Geometry check sheet. Reference: the model listing, model coordinates, mm. Face numbers are marked on the shaded views. A direction names the side the tool comes from. Give positions to 0.01 mm unless a question says otherwise; leave off trailing zeros. Write each loop counter-clockwise with the first axis right and the second up, starting at its lowest first coordinate (ties: lowest second). Pieces come first, ordered by that corner, then holes. Notation, with made-up numbers: (47, 81.25) - (90, 81.25) arc R7 ccw to (90, 86.25) - close; hole circle Ø2 at (36.5, 24.25). An arc over 180 degrees is marked (long way). Write item = value, one per line. Start each with the question number.
(1) Section check B-B, the plane y = -12. Enter the section's corners in (x, z), plus the area to 3 significant figures.
(2) Section check C-C, the plane z = 3. Enter the section's corners in (x, y).
(3) Section check A-A, the plane z = -10. Enter the section's corners in (x, y), plus the area to 3 significant figures.
(4) Access from +Z, -Z, +X, -X, +Y, -Y to the whole of each face (thin tool, end or side, straight path). Record for the marked faces 5 and 6.
(5) Draft check along X on the marked faces 1, 2, 3 and 4. Enter one of: pulls with the +X half, pulls with the -X half, needs draft (parallel to the pull), parting line crosses it, or undercut.
(6) Depth check by flat-ended pin: pin 1 Ø1.5 at (x, z) = (-1.5, -11) entering from +Y; pin 2 Ø8 at (x, y) = (8, 2) entering from -Z; pin 3 Ø4 at (x, z) = (10, -10) entering from +Y. Enter the tip coordinate at first touch or a pass-through.
(7) Thickness scan on L1, parallel to Z at x = -10, y = -12; L2, parallel to Z at x = 6.5, y = 2.25; L3, parallel to Y at x = -9, z = -14. Record the ranges inside material, lowest first.
(8) Section check D-D, the plane y = 0.75. Enter the section's corners in (x, z).
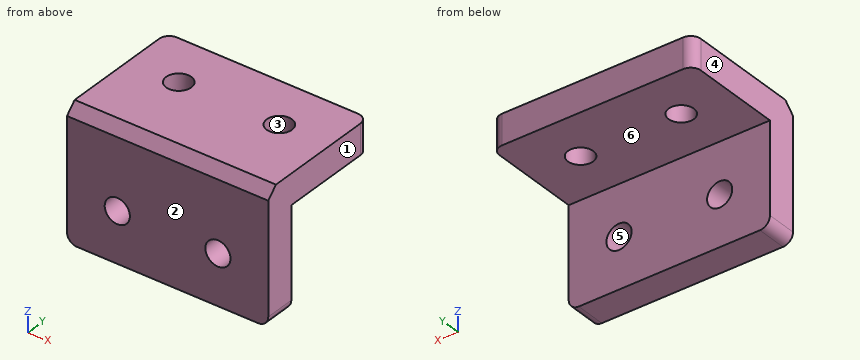
```python
from build123d import *

# Parameters (mm, degrees)
SKETCH1_R           = 2.5
BOSS_EXTRUDE2_DEPTH = 6
SKETCH3_W           = 40
SKETCH3_H           = 6
BOSS_EXTRUDE3_DEPTH = 26
SKETCH4_R           = 2.5
CUT_EXTRUDE2_DEPTH  = 26
CHAMFER1_SIZE       = 2


with BuildPart() as part:
    # Sketch1 → Boss-Extrude2 (new body)
    with BuildSketch(Plane.XY):
        with BuildLine():
            Line((-20, -9.25), (20, -9.25))
            Line((20, -9.25), (20, 8.75))
            ThreePointArc((20, 8.75), (19.414213562, 10.164213562), (18, 10.75))
            Line((18, 10.75), (-18, 10.75))
            ThreePointArc((-18, 10.75), (-19.414213562, 10.164213562), (-20, 8.75))
            Line((-20, 8.75), (-20, -9.25))
        make_face()
        with Locations((-10, 0.75)):
            Circle(SKETCH1_R, mode=Mode.SUBTRACT)
        with Locations((10, 0.75)):
            Circle(SKETCH1_R, mode=Mode.SUBTRACT)
    extrude(amount=BOSS_EXTRUDE2_DEPTH)

    # Sketch3 → Boss-Extrude3 (add)
    with BuildSketch(Plane.XY.offset(6)):
        with Locations((0, -12.25)):
            Rectangle(SKETCH3_W, SKETCH3_H)
    extrude(amount=-BOSS_EXTRUDE3_DEPTH)

    # Sketch4 → Cut-Extrude2 (cut)
    with BuildSketch(Plane.XZ.offset(15.25)):
        with Locations((-10, -10)):
            Circle(SKETCH4_R)
        with Locations((10, -10)):
            Circle(SKETCH4_R)
        with BuildLine():
            Line((-20, -20), (-18, -20))
            ThreePointArc((-18, -20), (-19.414213562, -19.414213562), (-20, -18))
            Line((-20, -18), (-20, -20))
        make_face()
        with BuildLine():
            ThreePointArc((20, -18), (19.414213562, -19.414213562), (18, -20))
            Line((18, -20), (20, -20))
            Line((20, -20), (20, -18))
        make_face()
    extrude(amount=-CUT_EXTRUDE2_DEPTH, mode=Mode.SUBTRACT)

    # Chamfer1
    chamfer1_edges = [part.edges().sort_by_distance(p)[0] for p in [
        (0, -15.25, 6),
    ]]
    chamfer(chamfer1_edges, length=CHAMFER1_SIZE)


solid = part.part
```
Model answer:
q1.outline = (-20, -18) arc R2 ccw to (-18, -20) - (18, -20) arc R2 ccw to (20, -18) - (20, 6) - (-20, 6) - close; hole circle Ø5 at (-10, -10); hole circle Ø5 at (10, -10)
q1.area = 999 mm²
q2.outline = (-20, -15.25) - (20, -15.25) - (20, 8.75) arc R2 ccw to (18, 10.75) - (-18, 10.75) arc R2 ccw to (-20, 8.75) - close; hole circle Ø5 at (-10, 0.75); hole circle Ø5 at (10, 0.75)
q3.outline = (-20, -15.25) - (-12.5, -15.25) - (-12.5, -9.25) - (-20, -9.25) - close; (-7.5, -15.25) - (7.5, -15.25) - (7.5, -9.25) - (-7.5, -9.25) - close; (12.5, -15.25) - (20, -15.25) - (20, -9.25) - (12.5, -9.25) - close
q3.area = 180 mm²
q4.face_5 = +Y, -Y
q4.face_6 = -Z, +X, -X, +Y
q5.face_1 = pulls with the +X half
q5.face_2 = needs draft
q5.face_3 = undercut
q5.face_4 = pulls with the -X half
q6.pin_1 = -9.25
q6.pin_2 = 0
q6.pin_3 = through
q7.L1 = -20 to -12.5, -7.5 to 6
q7.L2 = 0 to 6
q7.L3 = -15.25 to -9.25
q8.outline = (-20, 0) - (-12.5, 0) - (-12.5, 6) - (-20, 6) - close; (-7.5, 0) - (7.5, 0) - (7.5, 6) - (-7.5, 6) - close; (12.5, 0) - (20, 0) - (20, 6) - (12.5, 6) - close
